Geometry: final body of the model. Coordinates: model frame, mm. Face numbers are marked on the shaded views. A direction names the side the tool comes from. Give positions to 0.01 mm unless a question says otherwise; leave off trailing zeros. Write each loop counter-clockwise with the first axis right and the second up, starting at its lowest first coordinate (ties: lowest second). Pieces come first, ordered by that corner, then holes.
Q1. Pin query (flat end, axial travel): pin 1 (6 mm diameter, centred on x = -1.5, z = 79, fed in from -Y); pin 2 (1 mm diameter, centred on y = 25, z = 28, fed in from +X); pin 3 (6 mm diameter, centred on x = -25.5, z = 29.5, fed in from -Y). Return the tip coordinate at first contact, or that it passes through.
Q2. Cut plane A-A on x = 0. Return the cut outline in (y, z).
Q3. Line query: L1, parallel to Z at x = -3, y = -32.5; L2, parallel to Y at x = -1, z = 9.5; L3, parallel to X at y = 33, z = 39.5. Output: solid intervals per line, ascending.
Q4. Cut plane C-C on z = 32. Return the cut outline in (x, y), plus the area to 3 significant figures.
Q5. Reachability of the marked faces 1 and 2 from +Z, -Z, +X, -X, +Y, -Y: full face, straight path, thin tool, end or side. Return the list, or none.
```python
from build123d import *

# Parameters (mm, degrees)
F0_R     = 50
F1_DEPTH = 60
F2_R     = 5
F3_R     = 17.5
F4_DEPTH = 20
F5_R     = 7.5
F6_DEPTH = 10


with BuildPart() as f1:
    # F0 (on Top) → F1 (new body)
    with BuildSketch(Plane.XY):
        Circle(F0_R)
    extrude(amount=F1_DEPTH)

    # F2
    f2_edges = [f1.edges().sort_by_distance(p)[0] for p in [
        (-50, 0, 60),
        (-50, 0, 0),
    ]]
    fillet(f2_edges, radius=F2_R)

    # F3 (on face) → F4 (join)
    with BuildSketch(Plane.XY.offset(60)):
        Circle(F3_R)
    extrude(amount=F4_DEPTH)

    # F5 (on face) → F6 (join)
    with BuildSketch(Plane.XY.offset(80)):
        Circle(F5_R)
    extrude(amount=F6_DEPTH)


solid = f1.part
```
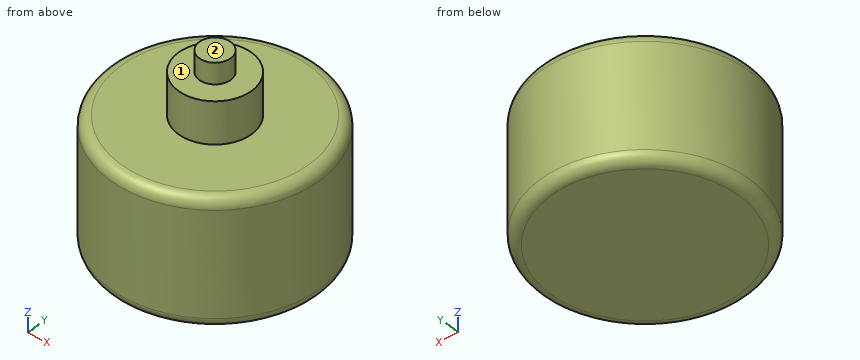
Data:
1. pin 1: stops at y = -17.5
1. pin 2: stops at x = 43.59
1. pin 3: stops at y = -44.65
2. outline: (-50, 5) arc R5 ccw to (-45, 0) - (45, 0) arc R5 ccw to (50, 5) - (50, 55) arc R5 ccw to (45, 60) - (17.5, 60) - (17.5, 80) - (7.5, 80) - (7.5, 90) - (-7.5, 90) - (-7.5, 80) - (-17.5, 80) - (-17.5, 60) - (-45, 60) arc R5 ccw to (-50, 55) - close
3. L1: z = 0 to 60
3. L2: y = -49.99 to 49.99
3. L3: x = -37.56 to 37.56
4. outline: circle Ø100 at (0, 0)
4. area: 7,850 mm2
5. face 1: +Z
5. face 2: +Z, +X, -X, +Y, -Y
